```python
from build123d import *

# Parameters (mm, degrees)
F0_W     = 1.6666666667
F0_H     = 1.6666666667
F2_DEPTH = 20
F1_R     = 10.75
F3_DEPTH = 5
F4_DEPTH = 1


with BuildPart() as f2:
    # F0 (on Top) → F2 (new body)
    with BuildSketch(Plane.XY):
        with Locations((0, 1.6666666667)):
            Rectangle(F0_W, F0_H)
        with Locations((-1.6666666667, 0)):
            Rectangle(F0_W, F0_H)
        with Locations((0, -1.6666666667)):
            Rectangle(F0_W, F0_H)
        Rectangle(F0_W, F0_H)
        with Locations((1.6666666667, 0)):
            Rectangle(F0_W, F0_H)
    extrude(amount=F2_DEPTH)



with BuildPart() as f3:
    # F1 (on Top) → F3 (new body)
    with BuildSketch(Plane.XY):
        Circle(F1_R)
        with BuildLine():
            ThreePointArc((-8.6602540538, 4.9999999724), (-5.0000000138, 8.6602540299), (0, 10))
            ThreePointArc((0, 10), (5.0000000138, 8.6602540299), (8.6602540538, 4.9999999724))
            ThreePointArc((8.6602540538, 4.9999999724), (9.659258267, 2.5881904356), (10, 0))
            ThreePointArc((10, 0), (9.6592582663, -2.5881904384), (8.6602540509, -4.9999999774))
            ThreePointArc((8.6602540509, -4.9999999774), (5.0000000086, -8.6602540329), (-6.2e-09, -10))
            ThreePointArc((-6.2e-09, -10), (-5.0000000165, -8.6602540283), (-8.6602540538, -4.9999999724))
            ThreePointArc((-8.6602540538, -4.9999999724), (-10, 0), (-8.6602540538, 4.9999999724))
        make_face(mode=Mode.SUBTRACT)
        with BuildLine():
            ThreePointArc((8.6602540538, 4.9999999724), (5.0000000138, 8.6602540299), (0, 10))
            ThreePointArc((0, 10), (-5.0000000138, 8.6602540299), (-8.6602540538, 4.9999999724))
            ThreePointArc((-8.6602540538, 4.9999999724), (-10, 0), (-8.6602540538, -4.9999999724))
            ThreePointArc((-8.6602540538, -4.9999999724), (-5.0000000165, -8.6602540283), (-6.2e-09, -10))
            ThreePointArc((-6.2e-09, -10), (5.0000000086, -8.6602540329), (8.6602540509, -4.9999999774))
            ThreePointArc((8.6602540509, -4.9999999774), (9.6592582663, -2.5881904384), (10, 0))
            ThreePointArc((10, 0), (9.659258267, 2.5881904356), (8.6602540538, 4.9999999724))
        make_face()
        with BuildLine():
            ThreePointArc((-5.3947095812, -4.125), (-6.6917762677, -5.8153702001), (-8.6602540538, -4.9999999724))
            ThreePointArc((-8.6602540538, -4.9999999724), (-7.5976428947, -2.4346297999), (-5.3947095812, -4.125))
        make_face(mode=Mode.SUBTRACT)
        with BuildLine():
            ThreePointArc((1.75, -8.25), (1.2374368649, -9.4874368693), (-6.2e-09, -10))
            ThreePointArc((-6.2e-09, -10), (-1.2374368649, -7.0125631307), (1.75, -8.25))
        make_face(mode=Mode.SUBTRACT)
        with BuildLine():
            ThreePointArc((8.8947095812, -4.125), (8.8350797806, -4.5779333163), (8.6602540509, -4.9999999774))
            ThreePointArc((8.6602540509, -4.9999999774), (5.4543393818, -3.6720666837), (8.8947095812, -4.125))
        make_face(mode=Mode.SUBTRACT)
        with BuildLine():
            ThreePointArc((-5.3947095812, 4.125), (-7.5976428947, 2.4346297999), (-8.6602540538, 4.9999999724))
            ThreePointArc((-8.6602540538, 4.9999999724), (-6.6917762677, 5.8153702001), (-5.3947095812, 4.125))
        make_face(mode=Mode.SUBTRACT)
        with BuildLine():
            ThreePointArc((1.75, 5.7391201416), (4.8218253805, 3.5707142143), (6, 0))
            ThreePointArc((6, 0), (-3.5707142143, -4.8218253805), (-1.75, 5.7391201416))
            Line((-1.75, 5.7391201416), (-1.75, 8))
            Line((-1.75, 8), (-1.7320508076, 8))
            ThreePointArc((-1.7320508076, 8), (-1.3228756555, 9.3956439237), (0, 10))
            ThreePointArc((0, 10), (1.2374368671, 9.4874368671), (1.75, 8.25))
            ThreePointArc((1.75, 8.25), (1.745506934, 8.1246782406), (1.7320508076, 8))
            Line((1.7320508076, 8), (1.75, 8))
            Line((1.75, 8), (1.75, 5.7391201416))
        make_face(mode=Mode.SUBTRACT)
        with BuildLine():
            ThreePointArc((8.8947095812, 4.125), (5.4543393811, 3.6720666865), (8.6602540538, 4.9999999724))
            ThreePointArc((8.6602540538, 4.9999999724), (8.8350797814, 4.5779333135), (8.8947095812, 4.125))
        make_face(mode=Mode.SUBTRACT)
    extrude(amount=F3_DEPTH)


with BuildPart() as f2_1:
    add(f2.part)

    add(f3.part)  # F4 merges F3
    # F1 (on Top) → F4 (join)
    with BuildSketch(Plane.XY):
        with BuildLine():
            ThreePointArc((-1.75, 5.7391201416), (-3.5707142143, -4.8218253805), (6, 0))
            ThreePointArc((6, 0), (4.8218253805, 3.5707142143), (1.75, 5.7391201416))
            ThreePointArc((1.75, 5.7391201416), (0, 6), (-1.75, 5.7391201416))
        make_face()
    extrude(amount=F4_DEPTH)


solid = f2_1.part
```
Verification items for the finished model (mm, model axes). A direction names the side the tool comes from. Round coordinates to 2 decimals unless told otherwise and drop trailing zeros. Write each loop counter-clockwise with the first axis right and the second up, starting at its lowest first coordinate (ties: lowest second). Pieces come first, ordered by that corner, then holes.
1. Access from +Z, -Z, +X, -X, +Y, -Y to the whole of each face (thin tool, end or side, straight path). Record for faces 4 (the flat face through (-1.75, 7, 2)), 5 (the flat face through (0, 0, 0)), 6 (the flat face through (-0.833, 2, 10)).
2. Section check C-C on x = -6.5. Enter the section's corners in (y, z).
3. Section check A-A on z = 3. Enter the section's corners in (x, y) (3 decimals), plus the area to 3 significant figures.
4. Scan lines: L1, parallel to X at y = 0.25, z = 2.75; L2, parallel to Y at x = 1.25, z = 3.5; L3, parallel to X at y = 2, z = 3.25. Record each from-to range of solid material in increasing order.
5. Section check B-B on y = -9.5. Enter the section's corners in (x, z), plus the area to 3 significant figures.
6. Section check D-D on y = 4.5. Enter the section's corners in (x, z), plus the area to 3 significant figures.
7. Gauge pin test, flat ends, axial feed: P1, Ø1.3, axis at x = 2, z = 15, coming from the -Y side; P2, Ø0.5, axis at x = 0, z = 10.5, coming from the -Y side; P3, Ø4, axis at x = -6.5, y = -3, coming from the +Z side. Record the tip position at first contact, or that the pin passes through.
8. Draft check along Y on faces 1 (the flat face through (2, 0.833, 10)), 2 (the flat face through (0.833, -2, 10)), 3 (the flat face through (0, 0, 20)). Enter one of: +Y half, -Y half, draft (parallel to the pull), parting line (faces both ways), or undercut.
Answer:
1. face 4: +Z, -Z
1. face 5: -Z, +X, -X, +Y, -Y
1. face 6: +Z
2. outline: (-8.56, 0) - (-5.75, 0) - (-5.75, 5) - (-8.56, 5) - close; (-2.5, 0) - (2.5, 0) - (2.5, 5) - (-2.5, 5) - close; (5.75, 0) - (8.56, 0) - (8.56, 5) - (5.75, 5) - close
3. outline: circle Ø21.5 at (0, 0); (-2.5, -0.833) - (-0.833, -0.833) - (-0.833, -2.5) - (0.833, -2.5) - (0.833, -0.833) - (2.5, -0.833) - (2.5, 0.833) - (0.833, 0.833) - (0.833, 2.5) - (-0.833, 2.5) - (-0.833, 0.833) - (-2.5, 0.833) - close; hole circle Ø3.5 at (-7.145, -4.125); hole circle Ø3.5 at (-7.145, 4.125); hole circle Ø3.5 at (0, -8.25); hole (-1.75, 5.739) arc R6 ccw (long way) to (1.75, 5.739) - (1.75, 8) - (1.732, 8) arc R1.75 ccw (long way) to (-1.732, 8) - (-1.75, 8) - close; hole circle Ø3.5 at (7.145, -4.125); hole circle Ø3.5 at (7.145, 4.125)
3. area: 203 mm2
4. L1: x = -10.75 to -5.99, -2.5 to 2.5, 5.99 to 10.75
4. L2: y = -10.68 to -9.47, -7.03 to -5.87, -0.83 to 0.83, 9.47 to 10.68
4. L3: x = -10.56 to -5.66, -0.83 to 0.83, 5.66 to 10.56
5. outline: (-5.03, 0) - (-1.22, 0) - (-1.22, 5) - (-5.03, 5) - close; (1.22, 0) - (5.03, 0) - (5.03, 5) - (1.22, 5) - close
5. area: 38.1 mm2
6. outline: (-9.76, 0) - (-8.85, 0) - (-8.85, 5) - (-9.76, 5) - close; (-5.44, 0) - (5.44, 0) - (5.44, 5) - (3.97, 5) - (3.97, 1) - (-3.97, 1) - (-3.97, 5) - (-5.44, 5) - close; (8.85, 0) - (9.76, 0) - (9.76, 5) - (8.85, 5) - close
6. area: 31.7 mm2
7. P1: stops at y = -0.83
7. P2: stops at y = -2.5
7. P3: stops at z = 5
8. face 1: undercut
8. face 2: undercut
8. face 3: draft
